Build history of the part. All positions in model axes, mm. A direction names the side the tool comes from. Coordinates: 2 decimals unless noted, no trailing zeros. Order: outer loops, then holes, each group sorted by start corner. A loop starts at its lowest first (then second) coordinate and runs counter-clockwise, first axis right, second up. Notation, with made-up numbers: (29, 83.25) -> (74, 83.25) arc R10 cw to (74, 99.25) -> close; hole circle Ø1 at (-40, 67). An arc over 180 degrees is marked (long way). Write each question's results on one line, items separated by ' | '.
Autodesk Inventor part; units mm, degrees
ref_plane "YZ Plane" through (0, 0, 0) normal (1, 0, 0) x (0, 1, 0)
ref_plane "XZ Plane" through (0, 0, 0) normal (0, 1, 0) x (-1, 0, 0)
ref_plane "XY Plane" through (0, 0, 0) normal (0, 0, 1) x (1, 0, 0)
sketch "Sketch1" plane through (0, 0, 0) normal (0, 1, 0) x (-1, 0, 0)
  line L0 (-28, 28) -> (28, 28)
  line L1 (28, 28) -> (28, -28)
  line L2 (28, -28) -> (-28, -28)
  line L3 (-28, -28) -> (-28, 28)
  line L4 (-28, 28) -> (28, -28) construction
  line L5 (28, 28) -> (-28, -28) construction
  point P0 (0, 0)
  dimension "d0" = 56
  dimension "d1" = 56
extrude "Extrusion1" add sketch "Sketch1" along normal blind 54.6
sketch "Sketch2" plane through (0, 54.6, 0) normal (0, 1, 0) x (1, 0, 0)
  circle A0 centre (0, 0) radius 19
  dimension "d4" = 38
extrude "Extrusion2" add sketch "Sketch2" along normal blind 1.5
sketch "Sketch3" plane through (0, 56.1, 0) normal (0, 1, 0) x (1, 0, 0)
  arc A0 (3.5, 1.9365) -> (3.5, -1.9365) centre (0, 0) ccw
  line L0 (3.5, -1.9365) -> (3.5, 1.9365)
  point P0 (4, 0)
  dimension "d7" = 8
  dimension "d8" = 0.5
extrude "Extrusion3" add sketch "Sketch3" along normal blind 19.5
properties part number "Linear Rail motor"
Item 1: Slice it at D-D, the plane z = -6. List the corners of the cut face in (x, y).
Answer:
outline: (-28, 0) -> (28, 0) -> (28, 54.6) -> (18.03, 54.6) -> (18.03, 56.1) -> (-18.03, 56.1) -> (-18.03, 54.6) -> (-28, 54.6) -> close
Item 2: Drill centre lines: line 1 (Y direction, x = -18.5, z = -24.5); line 2 (Y direction, x = 1.5, z = 7); line 3 (X direction, y = 55.5, z = 3.5). Where is each one in solid material? Low to high. Write a range as from..to.
Answer:
line 1: y = 0..54.6 | line 2: y = 0..56.1 | line 3: x = -18.67..18.67
Item 3: Tool access for faces 1 (the cylindrical face through (-4, 66, 0)), 2 (the flat face through (0, 0, 0)), 3 (the flat face through (3.5, 66, 0)): list every direction of +Z, -Z, +X, -X, +Y, -Y with a clear straight run to the whole face (end or side of a thin tool).
Answer:
face 1: +Y | face 2: +Z, -Z, +X, -X, -Y | face 3: +Z, -Z, +X, +Y
Item 4: Pin check, flat tips, straight feed: pin 1 (6 mm diameter, centred on x = 9, z = 6.5, fed in from +Y); pin 2 (5 mm diameter, centred on x = 19.5, z = -14.5, fed in from +Y); pin 3 (1.9 mm diameter, centred on y = 63.5, z = -0.5, fed in from +X). Stop position of each tip, or through.
Answer:
pin 1: stops at y = 56.1 | pin 2: stops at y = 54.6 | pin 3: stops at x = 3.5
Item 5: Slice it at A-A, the plane z = 0. List the corners of the cut face in (x, y), and give its area (3 significant figures).
Answer:
outline: (-28, 0) -> (28, 0) -> (28, 54.6) -> (19, 54.6) -> (19, 56.1) -> (3.5, 56.1) -> (3.5, 75.6) -> (-4, 75.6) -> (-4, 56.1) -> (-19, 56.1) -> (-19, 54.6) -> (-28, 54.6) -> close | area: 3,260 mm^2
Item 6: Slice it at C-C, the plane y = 62. List the corners of the cut face in (x, z).
Answer:
outline: (3.5, -1.94) -> (3.5, 1.94) arc R4 ccw (long way) to start
Item 7: Slice it at B-B, the plane x = 0. List the corners of the cut face in (y, z).
Answer:
outline: (0, -28) -> (54.6, -28) -> (54.6, -19) -> (56.1, -19) -> (56.1, -4) -> (75.6, -4) -> (75.6, 4) -> (56.1, 4) -> (56.1, 19) -> (54.6, 19) -> (54.6, 28) -> (0, 28) -> close
